```python
from build123d import *

# Parameters (mm, degrees)
BOSS_EXTRUDE1_DEPTH   = 20
SKETCH2_R             = 69.75
CUT_EXTRUDE1_DEPTH    = 10
SKETCH3_R             = 12.5
CUT_EXTRUDE2_DEPTH    = 210.276793028
SKETCH4_R             = 5
CUT_EXTRUDE3_DEPTH    = 210.992323907
CRVPATTERN2_OUTLINE_R = 5
CRVPATTERN2_DEPTH     = 20


# Read off the part's stored shape, not the designer's step: CrvPattern2
with BuildPart() as part:
    # Sketch1 → Boss-Extrude1 (new body)
    with BuildSketch(Plane.XY):
        with BuildLine():
            Line((0, 96), (89.69, 96))
            ThreePointArc((89.69, 96), (185.69, 0), (89.69, -96))
            Line((89.69, -96), (0, -96))
            ThreePointArc((0, -96), (-96, 0), (0, 96))
        make_face()
    extrude(amount=BOSS_EXTRUDE1_DEPTH)

    # Sketch2 → Cut-Extrude1 (cut)
    with BuildSketch(Plane.XY.offset(20)):
        with Locations((89.69, 0)):
            Circle(SKETCH2_R)
        Circle(SKETCH2_R)
    extrude(amount=-CUT_EXTRUDE1_DEPTH, mode=Mode.SUBTRACT)

    # Sketch3 → Cut-Extrude2 (cut, through all)
    with BuildSketch(Plane.XY.offset(10)):
        Circle(SKETCH3_R)
        with Locations((89.69, 0)):
            Circle(SKETCH3_R)
    extrude(amount=-CUT_EXTRUDE2_DEPTH, mode=Mode.SUBTRACT)

    # Sketch4 → Cut-Extrude3 (cut, through all)
    with BuildSketch(Plane.XY.offset(20)):
        with Locations((172.565, 0)):
            Circle(SKETCH4_R)
    extrude(amount=-CUT_EXTRUDE3_DEPTH, mode=Mode.SUBTRACT)

    # CrvPattern2 outline → CrvPattern2 (cut)
    with BuildSketch(Plane.XY):
        with Locations((162.039610622, 40.420285352)):
            Circle(CRVPATTERN2_OUTLINE_R)
        with Locations((162.039610622, -40.420285352)):
            Circle(CRVPATTERN2_OUTLINE_R)
        with Locations((133.136958542, -70.573560335)):
            Circle(CRVPATTERN2_OUTLINE_R)
        with Locations((93.198501794, -82.800700723)):
            Circle(CRVPATTERN2_OUTLINE_R)
        with Locations((44.845, -82.875)):
            Circle(CRVPATTERN2_OUTLINE_R)
        with Locations((-3.508501794, -82.800700723)):
            Circle(CRVPATTERN2_OUTLINE_R)
        with Locations((-43.446958542, -70.573560335)):
            Circle(CRVPATTERN2_OUTLINE_R)
        with Locations((-72.349610622, -40.420285352)):
            Circle(CRVPATTERN2_OUTLINE_R)
        with Locations((-82.875, 0)):
            Circle(CRVPATTERN2_OUTLINE_R)
        with Locations((-72.349610622, 40.420285352)):
            Circle(CRVPATTERN2_OUTLINE_R)
        with Locations((-43.446958542, 70.573560335)):
            Circle(CRVPATTERN2_OUTLINE_R)
        with Locations((-3.508501794, 82.800700723)):
            Circle(CRVPATTERN2_OUTLINE_R)
        with Locations((44.845, 82.875)):
            Circle(CRVPATTERN2_OUTLINE_R)
        with Locations((93.198501794, 82.800700723)):
            Circle(CRVPATTERN2_OUTLINE_R)
        with Locations((133.136958542, 70.573560335)):
            Circle(CRVPATTERN2_OUTLINE_R)
    extrude(amount=CRVPATTERN2_DEPTH, mode=Mode.SUBTRACT)


solid = part.part
```
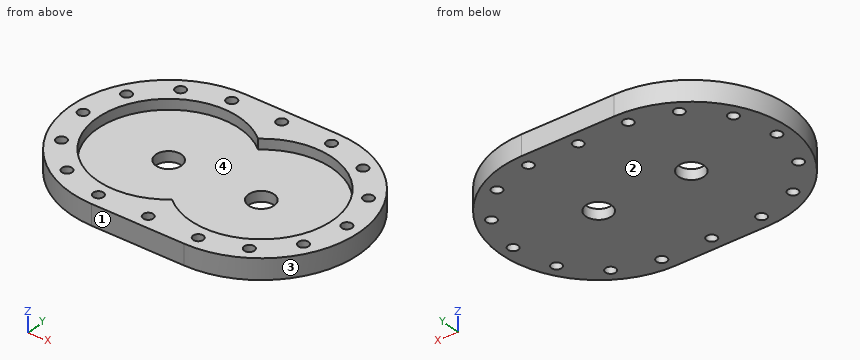
The model under review builds one solid part; all positions refer to its coordinate system, in mm. Face numbers are marked on the shaded views. Round coordinates to 2 decimals unless told otherwise and drop trailing zeros. Loops run counter-clockwise (first coordinate to the right, second up) from the corner with the lowest first, then second, coordinate; pieces in that order, holes last. Notation, with made-up numbers: M -22.5,33.25 L -6.5,33.25 A17 ccw -6.5,38.25 Z; hole C 43,33.5 d2. An arc over 180 degrees is marked long. Put each result on its own line as item: value.
Q1. Consider section B-B, the plane x = 9. Give the boundary of the cut face in (y, z).
Result set:
outline: M -96,0 L -8.67,0 L -8.67,10 L -69.17,10 L -69.17,20 L -96,20 Z; M 8.67,0 L 96,0 L 96,20 L 69.17,20 L 69.17,10 L 8.67,10 Z
Q2. Consider section C-C, the plane z = 14.25. Count the separate pieces of the cut face and the enclosed holes in it, then the cut area to 3 significant figures.
Result set:
separate pieces: 1
enclosed holes: 17
area: 18,000 mm²
Q3. Mouldability with a two-part tool opening along Y and no side actions: class the marked faces 1, 2, 3 and 4 as released by +Y, released by -Y, zero draft, split by the parting line, or undercut.
Result set:
face 1: released by -Y
face 2: zero draft
face 3: split by the parting line
face 4: undercut
Q4. For pin 1 (4 mm diameter, centred on x = 123.5, z = 13.5, fed in from -Y); pin 2 (6 mm diameter, centred on x = -3.51, y = 82.8, fed in from +Z); pin 3 (5 mm diameter, centred on x = 150, z = 14, fed in from +Y); pin 4 (1.5 mm diameter, centred on y = -73, z = 9, fed in from +X), all flat-tipped, find the tip position at first contact; note any pin that passes through.
Result set:
pin 1: stops at y = -90.58
pin 2: passes through
pin 3: stops at y = 76.64
pin 4: stops at x = 152.9
Q5. Consider section A-A, the plane y = 0. Give the boundary of the cut face in (x, z) (3 decimals), then the cut area to 3 significant figures.
Result set:
outline: M -96,0 L -87.875,0 L -87.875,20 L -96,20 Z; M -77.875,0 L -12.5,0 L -12.5,10 L -69.75,10 L -69.75,20 L -77.875,20 Z; M 12.5,0 L 77.19,0 L 77.19,10 L 12.5,10 Z; M 102.19,0 L 167.565,0 L 167.565,20 L 159.44,20 L 159.44,10 L 102.19,10 Z; M 177.565,0 L 185.69,0 L 185.69,20 L 177.565,20 Z
area: 2,440 mm²
Q6. Consider section D-D, the plane x = 108.5. Give the boundary of the cut face in (y, z), then the cut area to 3 significant figures.
Result set:
outline: M -94.14,0 L 94.14,0 L 94.14,20 L 67.17,20 L 67.17,10 L -67.17,10 L -67.17,20 L -94.14,20 Z
area: 2,420 mm²
Q7. To check wall thickness, follow L1, parallel to Y at x = 137, z = 4; L2, parallel to X at y = 10.5, z = 2.5; L3, parallel to Y at x = -44, z = 9.5. State the ranges of each line that lie inside material, in increasing order.
Result set:
L1: y = -83.53 to -73.75, -67.4 to 67.4, 73.75 to 83.53
L2: x = -95.42 to -6.78, 6.78 to 82.91, 96.47 to 185.11
L3: y = -85.32 to -75.54, -65.6 to 65.6, 75.54 to 85.32
